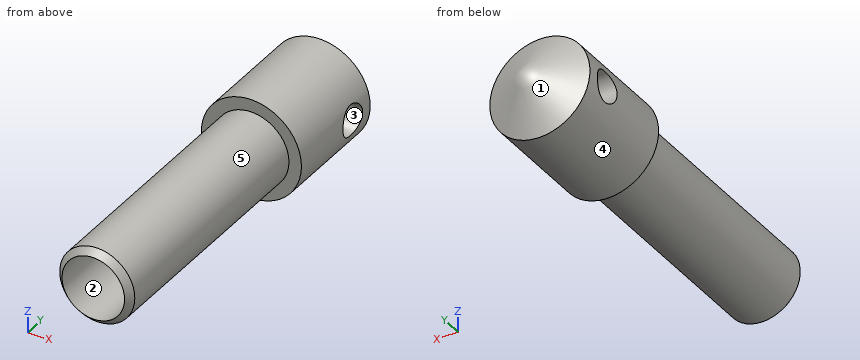
Autodesk Inventor part; units mm, degrees
ref_plane "YZ Plane" through (0, 0, 0) normal (1, 0, 0) x (0, 1, 0)
ref_plane "XZ Plane" through (0, 0, 0) normal (0, 1, 0) x (-1, 0, 0)
ref_plane "XY Plane" through (0, 0, 0) normal (0, 0, 1) x (1, 0, 0)
sketch "草圖1" plane through (0, 0, 0) normal (0, 0, 1) x (1, 0, 0)
  line L0 (0, 0) -> (6, 0)
  line L1 (6, 0) -> (6, 40)
  line L2 (6, 40) -> (8, 40)
  line L3 (8, 40) -> (8, 57.3812)
  line L4 (0, 62) -> (0, 64.8191)
  line L5 (0, 62) -> (8, 57.3812)
  line L6 (0, 0) -> (0, 62)
  dimension "d0" = 6
  dimension "d1" = 40
  dimension "d3" = 2
  dimension "d6" = 60
  dimension "d7" = 0
  dimension "d8" = 62
revolve "迴轉1" add sketch "草圖1" angle 360 about axis through (0, 62, 0) along (0, 1, 0)
chamfer "倒角1" distance 1 distance2 1 1 edges at (-6, 0, 0) measured on face at (-3.0269, 0, 1.5886)
sketch "草圖2" plane through (0, 0, 0) normal (0, -1, 0) x (1, 0, 0)
  circle A0 centre (0, 0) radius 5
extrude "擠出1" cut sketch "草圖2" against normal blind 36
sketch "草圖4" plane through (0, 0, 0) normal (1, 0, 0) x (0, 1, 0)
  circle A0 centre (53, 0) radius 2.5
  line L0 (40, 8) -> (40, -8)
  point P0 (0, 0)
  dimension "d17" = 13
  dimension "d18" = 5
  dimension "d19" = 0
extrude "擠出2" cut sketch "草圖4" along normal through all both and the other way through all
thread "螺紋2"
thread "螺紋3"
properties part number "B"
Model file for the job. Use its own axes, mm. Face numbers are marked on the shaded views. A direction names the side the tool comes from. Give positions to 0.01 mm unless a question says otherwise; leave off trailing zeros. Loops run counter-clockwise (first coordinate to the right, second up) from the corner with the lowest first, then second, coordinate; pieces in that order, holes last. Notation, with made-up numbers: (69.25, -18) -> (73.25, -18) arc R31 ccw to (73.25, 17) -> close; hole circle Ø5 at (-36, 49.5). An arc over 180 degrees is marked (long way). Use a Markdown table: item, result. Add a question column.
(1) Wall check: line 1 along X through (y, z) = (25.5, 0); line 2 along Y through (x, z) = (-2.75, -0.5). Give the ranges that are in metal, low to high.
(2) Slice it at B-B on y = 53. List the corners of the cut face in (x, z).
(3) Mould opens along Y. For the marked faces 1, 2 and 3 say: +Y half, -Y half, draft (parallel to the pull), parting line (faces both ways), or undercut.
(4) Tool access for the marked faces 4 and 5: list every direction of +Z, -Z, +X, -X, +Y, -Y with a clear straight run to the whole face (end or side of a thin tool).
(5) Slice it at A-A on y = 6.5. List the corners of the cut face in (x, z), and give its area (3 significant figures).
(6) Drop flat-ended pins along their axis: pin 1 Ø4.5 at (y, z) = (53, 0) entering from -X; pin 2 Ø6 at (x, z) = (5, 1.5) entering from -Y; pin 3 Ø3 at (y, z) = (42.5, -3.5) entering from -X; pin 4 Ø5 at (x, z) = (1, -1) entering from -Y. Give the stop position or say it passes through.
Filled sheet:
| question | item | result |
|---|---|---|
| 1 | line 1 | -6 to -5, 5 to 6 |
| 1 | line 2 | 36 to 50.55, 55.45 to 60.39 |
| 2 | outline | (-7.6, -2.5) arc R8 ccw to (7.6, -2.5) -> close; (-7.6, 2.5) -> (7.6, 2.5) arc R8 ccw to start |
| 3 | face 1 | +Y half |
| 3 | face 2 | draft |
| 3 | face 3 | undercut |
| 4 | face 4 | +Y, -Y |
| 4 | face 5 | -Y |
| 5 | outline | circle Ø12 at (0, 0); hole circle Ø10 at (0, 0) |
| 5 | area | 34.6 mm2 |
| 6 | pin 1 | through |
| 6 | pin 2 | y = 0 |
| 6 | pin 3 | x = -7.75 |
| 6 | pin 4 | y = 36 |
